from build123d import *

# Parameters (mm, degrees)
SKETCH1_R           = 1.1811
BOSS_EXTRUDE1_DEPTH = 25.4
FILLET2_R           = 0.254
SKETCH2_R           = 2.4638
CUT_EXTRUDE1_DEPTH  = 8.72109
SKETCH3_R           = 2.4638
CUT_EXTRUDE2_DEPTH  = 8.72109
SKETCH5_W           = 1.7273194
SKETCH5_H           = 1.763863254
CUT_EXTRUDE3_DEPTH  = 8.72109
SKETCH6_W           = 1.964621561
SKETCH6_H           = 1.893145227
CUT_EXTRUDE4_DEPTH  = 8.72109
FILLET3_R           = 0.254
FILLET4_R           = 0.254
SKETCH7_R           = 1.7907
CUT_EXTRUDE5_DEPTH  = 2.54


with BuildPart() as part:
    # Sketch1 → Boss-Extrude1 (new body)
    with BuildSketch(Plane.XY):
        with BuildLine():
            Line((-17.6276, 2.614576368), (-17.6276, 3.884576368))
            Line((-17.6276, 3.884576368), (-7.224163794, 3.884576368))
            ThreePointArc((-7.224163794, 3.884576368), (-3.076448638, 6.402723098), (-6.1087, 2.614576368))
            Line((-6.1087, 2.614576368), (-17.6276, 2.614576368))
        make_face()
        with Locations((-4.9276, 4.776823632)):
            Circle(SKETCH1_R, mode=Mode.SUBTRACT)
    extrude(amount=BOSS_EXTRUDE1_DEPTH)

    # Fillet2
    fillet2_edges = [part.edges().sort_by_distance(p)[0] for p in [
        (-7.224163794, 3.884576368, 12.7),
    ]]
    fillet(fillet2_edges, radius=FILLET2_R)

    # Sketch2 → Cut-Extrude1 (cut)
    with BuildSketch(Plane(origin=(0, 0, 0), x_dir=(-1, 0, 0), z_dir=(0, 0, -1))):
        with Locations((4.9276, 4.776823632)):
            Circle(SKETCH2_R)
    extrude(amount=-CUT_EXTRUDE1_DEPTH, mode=Mode.SUBTRACT)

    # Sketch3 → Cut-Extrude2 (cut)
    with BuildSketch(Plane.XY.offset(25.4)):
        with Locations((-4.9276, 4.776823632)):
            Circle(SKETCH3_R)
    extrude(amount=-CUT_EXTRUDE2_DEPTH, mode=Mode.SUBTRACT)

    # Sketch5 → Cut-Extrude3 (cut)
    with BuildSketch(Plane(origin=(0, 0, 0), x_dir=(-1, 0, 0), z_dir=(0, 0, -1))):
        with Locations((6.7817403, 3.496507995)):
            Rectangle(SKETCH5_W, SKETCH5_H)
    extrude(amount=-CUT_EXTRUDE3_DEPTH, mode=Mode.SUBTRACT)

    # Sketch6 → Cut-Extrude4 (cut)
    with BuildSketch(Plane.XY.offset(25.4)):
        with Locations((-6.663089219, 3.561148982)):
            Rectangle(SKETCH6_W, SKETCH6_H)
    extrude(amount=-CUT_EXTRUDE4_DEPTH, mode=Mode.SUBTRACT)

    # Fillet3
    fillet3_edges = [part.edges().sort_by_distance(p)[0] for p in [
        (-7.6454, 3.249576368, 16.67891),
    ]]
    fillet(fillet3_edges, radius=FILLET3_R)

    # Fillet4
    fillet4_edges = [part.edges().sort_by_distance(p)[0] for p in [
        (-7.6454, 3.249576368, 8.72109),
    ]]
    fillet(fillet4_edges, radius=FILLET4_R)

    # Sketch7 → Cut-Extrude5 (cut)
    with BuildSketch(Plane(origin=(0, 3.884576368, 0), x_dir=(1, 0, 0), z_dir=(0, 1, 0))):
        with Locations((-12.6365, -4.8514)):
            Circle(SKETCH7_R)
        with Locations((-12.6365, -20.5486)):
            Circle(SKETCH7_R)
    extrude(amount=-CUT_EXTRUDE5_DEPTH, mode=Mode.SUBTRACT)


solid = part.part
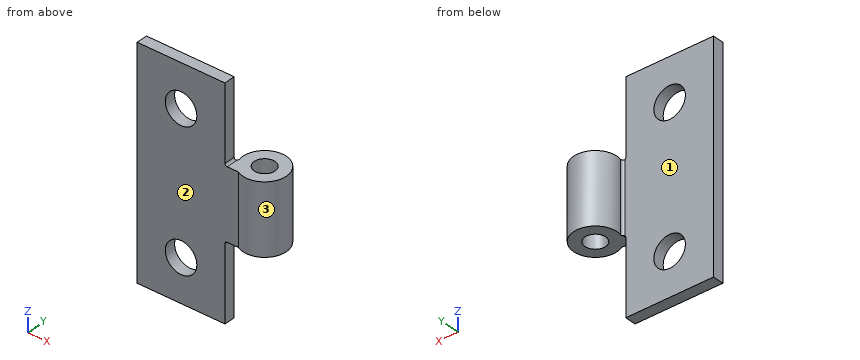
Read the model definition and answer for the solid it produces. Units are mm, in the model's axes. Face numbers are marked on the shaded views. A direction names the side the tool comes from. Round coordinates to 2 decimals unless told otherwise and drop trailing zeros. Order: outer loops, then holes, each group sorted by start corner. A loop starts at its lowest first (then second) coordinate and runs counter-clockwise, first axis right, second up.
1) The part is cut by section B-B on x = -14. Write down the section's boundary in (y, z).
2) The part is cut by section A-A on y = 4.45. Write down the section's boundary in (x, z).
3) The part is cut by section C-C on z = 5.75. Write down the section's boundary in (x, y), plus the area to 3 significant figures.
4) Flat-ended cylindrical pins translate along their axes: pin 1 (1 mm diameter, centred on x = -13.5, z = 7.5, fed in from -Y); pin 2 (1.5 mm diameter, centred on x = -4, y = 5, fed in from +Z); pin 3 (3 mm diameter, centred on x = -15.5, z = 8, fed in from +Y); pin 4 (1.4 mm diameter, centred on x = -4.93, y = 4.78, fed in from -Z). Find the tip coordinate at first contact, or state that the pin passes through.
5) For the marked faces 1, 2 and 3, determine the directions among +Z, -Z, +X, -X, +Y, -Y from which every point of the face is accessible in a straight line to the end or side of a thin tool.
6) Straight lines are drawn through the part: L1, parallel to Y at x = -16.75, z = 6.75; L2, parallel to X at y = 3.2, z = 2.5; L3, parallel to Y at x = -5.25, z = 11.5. For each, find the intervals that lie inside material, in ascending order.
7) The part is cut by section D-D on y = 3.2. Write down the section's boundary in (x, z).
Resolved:
1. outline: (2.61, 0) - (3.88, 0) - (3.88, 3.69) - (2.61, 3.69) - close; (2.61, 6.01) - (3.88, 6.01) - (3.88, 19.39) - (2.61, 19.39) - close; (2.61, 21.71) - (3.88, 21.71) - (3.88, 25.4) - (2.61, 25.4) - close
2. outline: (-7.37, 8.72) - (-6.06, 8.72) - (-6.06, 16.68) - (-7.37, 16.68) - close; (-3.79, 8.72) - (-2.49, 8.72) - (-2.49, 16.68) - (-3.79, 16.68) - close
3. outline: (-17.63, 2.61) - (-14.19, 2.61) - (-14.19, 3.88) - (-17.63, 3.88) - close; (-11.09, 2.61) - (-7.65, 2.61) - (-7.65, 3.88) - (-11.09, 3.88) - close
3. area: 8.74 mm2
4. pin 1: stops at y = 2.61
4. pin 2: stops at z = 16.68
4. pin 3: stops at y = 3.88
4. pin 4: passes through
5. face 1: +Z, -Z, -X, +Y
5. face 2: +Z, -Z, -X, -Y
5. face 3: +Z, -Z
6. L1: y = 2.61 to 3.88
6. L2: x = -17.63 to -7.65
6. L3: y = 2.33 to 3.64, 5.91 to 7.22
7. outline: (-17.63, 0) - (-7.65, 0) - (-7.65, 8.47) arc R0.25 cw to (-7.39, 8.72) - (-3.03, 8.72) - (-3.03, 16.68) - (-7.39, 16.68) arc R0.25 cw to (-7.65, 16.93) - (-7.65, 25.4) - (-17.63, 25.4) - close; hole circle Ø3.58 at (-12.64, 4.85); hole circle Ø3.58 at (-12.64, 20.55)
